Read the model definition and answer for the solid it produces. Units are mm, in the model's axes. A direction names the side the tool comes from. Give positions to 0.01 mm unless a question says otherwise; leave off trailing zeros. Write each loop counter-clockwise with the first axis right and the second up, starting at its lowest first coordinate (ties: lowest second). Pieces come first, ordered by that corner, then holes. Notation, with made-up numbers: (44, -20.5) - (102, -20.5) arc R34 cw to (102, 16.5) - close; hole circle Ø11 at (15.5, 53). An arc over 180 degrees is marked (long way). Use CSV: the item, a comma, the result in double quotes. Start each with the question number.
Autodesk Fusion 360 part; units mm, degrees
sketch "Sketch1" plane through (0, 0, 0) normal (0, 0, 1) x (1, 0, 0)
  line L0 (9.9, 9.9) -> (-9.9, 9.9)
  line L1 (-9.9, 9.9) -> (-9.9, -9.9)
  line L2 (-9.9, -9.9) -> (9.9, -9.9)
  line L3 (9.9, -9.9) -> (9.9, 9.9)
  line L4 (9.9, 9.9) -> (-9.9, -9.9) construction
  line L5 (-9.9, 9.9) -> (9.9, -9.9) construction
  line L6 (11, -11) -> (-11, -11)
  line L7 (-11, -11) -> (-11, 11)
  line L8 (-11, 11) -> (11, 11)
  line L9 (11, 11) -> (11, -11)
  line L10 (11, -11) -> (-11, 11) construction
  line L11 (-11, -11) -> (11, 11) construction
  line L12 (8.9, -8.9) -> (-8.9, -8.9)
  line L13 (-8.9, -8.9) -> (-8.9, 8.9)
  line L14 (-8.9, 8.9) -> (8.9, 8.9)
  line L15 (8.9, 8.9) -> (8.9, -8.9)
  line L16 (8.9, -8.9) -> (-8.9, 8.9) construction
  line L17 (-8.9, -8.9) -> (8.9, 8.9) construction
  line L18 (8.4, -6) -> (-8.4, -6)
  line L19 (-8.4, -6) -> (-8.4, 6)
  line L20 (-8.4, 6) -> (8.4, 6)
  line L21 (8.4, 6) -> (8.4, -6)
  line L22 (8.4, -6) -> (-8.4, 6) construction
  line L23 (-8.4, -6) -> (8.4, 6) construction
  line L24 (8.0957, 8.0957) -> (-8.0957, 8.0957)
  line L25 (-8.0957, 8.0957) -> (-8.0957, -8.0957)
  line L26 (-8.0957, -8.0957) -> (8.0957, -8.0957)
  line L27 (8.0957, -8.0957) -> (8.0957, 8.0957)
  line L28 (8.0957, 8.0957) -> (-8.0957, -8.0957) construction
  line L29 (-8.0957, 8.0957) -> (8.0957, -8.0957) construction
  line L30 (8.9, -0.5) -> (-8.9, -0.5)
  line L31 (-8.9, -0.5) -> (-8.9, 0.5)
  line L32 (-8.9, 0.5) -> (8.9, 0.5)
  line L33 (8.9, 0.5) -> (8.9, -0.5)
  line L34 (8.9, -0.5) -> (-8.9, 0.5) construction
  line L35 (-8.9, -0.5) -> (8.9, 0.5) construction
  dimension "d1" = 19.8
  dimension "d2" = 19.8
  dimension "d3" = 22
  dimension "d4" = 22
  dimension "d5" = 17.8
  dimension "d6" = 17.8
  dimension "d7" = 16.8
  dimension "d8" = 12
  dimension "d53" = 1
extrude "Extrude1" add sketch "Sketch1" along normal blind 1 contours L12 L13 L15 L18 L19 L21 L25 L26 L27 L30 | L15 L21 L30 L32 L33 | L13 L19 L30 L31 L32 | L13 L14 L15 L19 L20 L21 L24 L25 L27 L32 | L18 L25 L26 L27 | L20 L24 L25 L27
extrude "Extrude2" add sketch "Sketch1" along normal blind 4 contours L0 L1 L2 L3
extrude "Extrude3" add sketch "Sketch1" along normal blind 5 contours L6 L7 L8 L9
extrude "Extrude4" cut sketch "Sketch1" along normal blind 4 contours L6 L7 L8 L9
extrude "Extrude5" add 1 faces at (-9.5667, -2.9667, 4) along direction (0, 0, 1) blind 1
fillet "Fillet1" radius 3 1 edges at (9.9, -9.9, 2)
fillet "Fillet2" radius 3 1 edges at (-9.9, -9.9, 2)
fillet "Fillet3" radius 3 2 edges at (-9.9, 9.9, 2) (9.9, 9.9, 2)
fillet "Fillet4" radius 1 4 edges at (-11, -11, 4.5) (-11, 11, 4.5) (11, -11, 4.5) (11, 11, 4.5)
extrude "Extrude6" add 1 faces at (-2.8, -7.9333, 1) along direction (0, 0, 1) blind 5
extrude "Extrude7" cut sketch "Sketch1" along normal blind 3 contours L18 L25 L26 L27 | L20 L24 L25 L27
extrude "Extrude8" cut 1 faces at (-8.0957, 7.3972, 1) along direction (-1, 0, 0) blind 0.304
extrude "Extrude9" cut 1 faces at (8.0957, 6.6986, 1) along direction (1, 0, 0) blind 0.304
extrude "Extrude10" cut 1 faces at (8.0957, -7.3972, 1) along direction (1, 0, 0) blind 0.304
extrude "Extrude11" cut 1 faces at (-8.0957, -6.6986, 1) along direction (-1, 0, 0) blind 0.304
sketch "Sketch2" plane through (8.4, 0, 0) normal (-1, 0, 0) x (0, -1, 0)
  line L0 (-6, 0) -> (6, 0)
  line L1 (6, 0) -> (6, 6)
  line L2 (6, 6) -> (-6, 6)
  line L3 (-6, 6) -> (-6, 0)
  line L4 (-6, 6) -> (6, 6)
  line L5 (6, 6) -> (6, 4.0166)
  line L6 (6, 4.0166) -> (-6, 4.0166)
  line L7 (-6, 4.0166) -> (-6, 6)
extrude "Extrude12" add sketch "Sketch2" along normal blind 1 contours L1 L2 L3 L4 L5 L6 L7
sketch "Sketch3" plane through (-8.4, 0, 0) normal (1, 0, 0) x (0, 1, 0)
  line L0 (-6, 0) -> (6, 0)
  line L1 (6, 0) -> (6, 6)
  line L2 (6, 6) -> (-6, 6)
  line L3 (-6, 6) -> (-6, 0)
  line L4 (-6, 6) -> (6, 6)
  line L5 (6, 6) -> (6, 3.9624)
  line L6 (6, 3.9624) -> (-6, 3.9624)
  line L7 (-6, 3.9624) -> (-6, 6)
extrude "Extrude13" add sketch "Sketch3" along normal blind 1 contours L1 L2 L3 L4 L5 L6 L7
extrude "Extrude14" cut 1 faces at (-2.4667, 7.9333, 6) along direction (0, 0, -1) blind 2
extrude "Extrude15" add 1 faces at (-2.4667, 7.9333, 4) along direction (0, 0, 1) blind 1
sketch "TOP BUTTON GUIDE" plane through (0, 0, 5) normal (0, 0, 1) x (-1, 0, 0)
  line L0 (-8.4, 6) -> (7.4, 6)
  line L1 (7.4, 6) -> (7.4, -6)
  line L2 (7.4, -6) -> (-8.4, -6)
  line L3 (-8.4, -6) -> (-8.4, 6)
  arc A0 (-11, -10) -> (-10, -11) centre (-10, -10) ccw
  line L4 (-10, -11) -> (10, -11)
  arc A1 (10, -11) -> (11, -10) centre (10, -10) ccw
  line L5 (11, -10) -> (11, 10)
  arc A2 (11, 10) -> (10, 11) centre (10, 10) ccw
  line L6 (10, 11) -> (-10, 11)
  arc A3 (-10, 11) -> (-11, 10) centre (-10, 10) ccw
  line L7 (-11, 10) -> (-11, -10)
  line L8 (-8.35, 8.25) -> (8.35, 8.25)
  line L9 (8.35, 8.25) -> (8.35, -8.25)
  line L10 (8.35, -8.25) -> (-8.35, -8.25)
  line L11 (-8.35, -8.25) -> (-8.35, 8.25)
  line L12 (-8.35, 8.25) -> (8.35, -8.25) construction
  line L13 (8.35, 8.25) -> (-8.35, -8.25) construction
  line L14 (-9.15, 9.05) -> (9.15, 9.05)
  line L15 (9.15, 9.05) -> (9.15, -9.05)
  line L16 (9.15, -9.05) -> (-9.15, -9.05)
  line L17 (-9.15, -9.05) -> (-9.15, 9.05)
  line L18 (-9.15, 9.05) -> (9.15, -9.05) construction
  line L19 (9.15, 9.05) -> (-9.15, -9.05) construction
  dimension "d47" = 16.7
  dimension "d48" = 16.5
  dimension "d49" = 18.3
  dimension "d50" = 18.1
extrude "Extrude16" add sketch "TOP BUTTON GUIDE" along normal blind 2 contours L14 L15 L16 L17
extrude "Extrude17" add sketch "Sketch1" along normal blind 5 contours L21 L27 L30 L32 | L19 L25 L30 L32 | L25 L27 L30 L32
sketch "Sketch5" plane through (0, 0, 5) normal (0, 0, 1) x (-1, 0, 0)
  line L0 (7.4, -0.5) -> (7.4, -6)
  line L1 (7.4, -6) -> (-8.35, -6)
  line L2 (-8.35, -6) -> (-8.35, -8.25)
  line L3 (-8.35, -8.25) -> (8.35, -8.25)
  line L4 (8.35, -8.25) -> (8.35, 8.25)
  line L5 (8.35, 8.25) -> (-8.35, 8.25)
  line L6 (-8.35, 8.25) -> (-8.35, 6)
  line L7 (-8.35, 6) -> (7.4, 6)
  line L8 (7.4, 6) -> (7.4, 0.5)
  line L9 (7.4, 0.5) -> (-8.4, 0.5)
  line L10 (-8.4, 0.5) -> (-8.4, -0.5)
  line L11 (-8.4, -0.5) -> (7.4, -0.5)
  line L12 (-3.5, 1.3147) -> (3.5, 1.3147)
  line L13 (3.5, 1.3147) -> (3.5, -1.3147)
  line L14 (3.5, -1.3147) -> (-3.5, -1.3147)
  line L15 (-3.5, -1.3147) -> (-3.5, 1.3147)
  line L16 (-3.5, 1.3147) -> (3.5, -1.3147) construction
  line L17 (3.5, 1.3147) -> (-3.5, -1.3147) construction
  dimension "d56" = 7
extrude "Extrude18" cut sketch "Sketch5" against normal blind 6 contours L9 L11 L13 L15
extrude "Extrude19" cut 1 faces at (-2.7833, 8.25, 5.6667) along direction (0, 1, 0) blind 0.5
extrude "Extrude20" add 1 faces at (-3.05, 9.05, 5.6667) along direction (0, 1, 0) blind 0.5
extrude "Extrude21" cut 1 faces at (-8.35, 3.0833, 6.3333) along direction (-1, 0, 0) blind 0.3
extrude "Extrude22" add 1 faces at (-9.15, 3.35, 5.6667) along direction (-1, 0, 0) blind 0.3
sketch "Sketch6" plane through (0, 0, 5) normal (0, 0, 1) x (-1, 0, 0)
  line L0 (3.5, 0.5) -> (3.5, -0.5)
  line L1 (3.5, -0.5) -> (7.4, -0.5)
  line L2 (7.4, -0.5) -> (7.4, -6)
  line L3 (7.4, -6) -> (-8.35, -6)
  line L4 (-8.35, -6) -> (-8.35, -8.75)
  line L5 (-8.35, -8.75) -> (8.65, -8.75)
  line L6 (8.65, -8.75) -> (8.65, 8.25)
  line L7 (8.65, 8.25) -> (-8.35, 8.25)
  line L8 (-8.35, 8.25) -> (-8.35, 6)
  line L9 (-8.35, 6) -> (7.4, 6)
  line L10 (7.4, 6) -> (7.4, 0.5)
  line L11 (7.4, 0.5) -> (3.5, 0.5)
  circle A0 centre (6.4473, -6.6661) radius 0.4424
extrude "Extrude23" cut sketch "Sketch6" against normal blind 2 contours A0
extrude "Extrude24" cut 1 faces at (-3.5, -0.1667, 3.3333) along direction (-1, 0, 0) blind 0.6
extrude "Extrude25" cut 1 faces at (3.5, 0.1667, 3.3333) along direction (1, 0, 0) blind 0.6
extrude "Extrude26" add 1 faces at (-9.1833, -2.5833, 7) along direction (0, 0, 1) blind 5
extrude "Extrude27" cut 1 faces at (-9.1833, -2.5833, 12) along direction (0, 0, -1) blind 2
(1) The part is cut by section A-A on y = -3. Write down the section's boundary in (x, z), plus the area to 3 significant figures.
(2) The part is cut by section C-C on x = 6.5. Write down the section's boundary in (y, z).
(3) Which of the six approach directions +Z, -Z, +X, -X, +Y, -Y give full straight-line access (tool end or side, diameter ignored) to faces 1 (the face through (-4.1, 0, 3)), 2 (the face through (9.9, 0, 2)), 3 (the face through (0, -9.05, 7)), 4 (the face through (-8, 3, 3.962)), 5 (the face through (0, -9.9, 2))?
(4) Consider probe 1 along Y at (x, z) = (-5.75, 1.5); probe 2 along Y at (x, z) = (-1.25, 1); probe 3 along Y at (x, z) = (-4.25, 6). Determine where each line is inside the solid, lowest interval first.
(5) For a pull along Y with two mould halves and no side action, classify faces 6 (the face through (-8.4, 3, 2)), 7 (the face through (0, 8.096, 1)), 8 (the face through (10.715, 10.699, 4.507)), 9 (the face through (-5, 0, 0)) as pulls with the +Y half, pulls with the -Y half, needs draft (parallel to the pull), parting line crosses it, or undercut.
(6) Given P1, Ø11, axis at x = 1.5, y = 1.5, coming from the +Z side; P2, Ø2.5, axis at y = -7, z = 1, coming from the -X side; P3, Ø3, axis at x = 3, y = 6, coming from the -Z side; P4, Ø6, axis at y = 0, z = 7, coming from the -X side, each flat-ended and moving along its own axis, determine where each tip first touches the part or whether it passes through.
(7) The part is cut by section D-D on x = 0.5. Write down the section's boundary in (y, z), plus the area to 3 significant figures.
Reported:
1,outline,"(-11, 4) - (-9.9, 4) - (-9.9, 0) - (-8.4, 0) - (-8.4, 3.96) - (-7.4, 3.96) - (-7.4, 5) - (-8.65, 5) - (-8.65, 10) - (-9.45, 10) - (-9.45, 5) - (-11, 5) - close; (8.4, 0) - (9.9, 0) - (9.9, 4) - (11, 4) - (11, 5) - (9.15, 5) - (9.15, 10) - (8.4, 10) - close"
1,area,"26.0 mm²"
2,outline,"(-11, 4) - (-9.9, 4) - (-9.9, 0) - (-8.1, 0) - (-8.1, 3) - (-6, 3) - (-6, 5) - (-8.25, 5) - (-8.25, 10) - (-9.05, 10) - (-9.05, 5) - (-11, 5) - close; (-0.5, 0) - (0.5, 0) - (0.5, 5) - (-0.5, 5) - close; (6, 3) - (8.1, 3) - (8.1, 0) - (9.9, 0) - (9.9, 4) - (11, 4) - (11, 5) - (9.55, 5) - (9.55, 10) - (8.75, 10) - (8.75, 5) - (6, 5) - close"
3,face 1,"+Z, -Z"
3,face 2,"-Z, +X, +Y, -Y"
3,face 3,"+Z, +X, -X, -Y"
3,face 4,"-Z"
3,face 5,"-Z, +X, -X, -Y"
4,probe 1,"-9.9 to -8.1, -0.5 to 0.5, 8.1 to 9.9"
4,probe 2,"-9.9 to -8.1, 8.1 to 9.9"
4,probe 3,"-9.05 to -8.25, 8.75 to 9.55"
5,face 6,"undercut"
5,face 7,"undercut"
5,face 8,"pulls with the +Y half"
5,face 9,"needs draft"
6,P1,"z = 5"
6,P2,"x = -9.9"
6,P3,"z = 3"
6,P4,"x = -11"
7,outline,"(-11, 4) - (-9.9, 4) - (-9.9, 0) - (-8.1, 0) - (-8.1, 3) - (-6, 3) - (-6, 5) - (-8.25, 5) - (-8.25, 10) - (-9.05, 10) - (-9.05, 5) - (-11, 5) - close; (6, 3) - (8.1, 3) - (8.1, 0) - (9.9, 0) - (9.9, 4) - (11, 4) - (11, 5) - (9.55, 5) - (9.55, 10) - (8.75, 10) - (8.75, 5) - (6, 5) - close"
7,area,"36.6 mm²"
